CAD build for the part. Positions are in the model's coordinates, mm. A direction names the side the tool comes from. Give positions to 0.01 mm unless a question says otherwise; leave off trailing zeros. Write each loop counter-clockwise with the first axis right and the second up, starting at its lowest first coordinate (ties: lowest second). Pieces come first, ordered by that corner, then holes. Notation, with made-up numbers: (41.5, 30) - (54.5, 30) arc R17 ccw to (54.5, 58) - close; hole circle Ø11 at (54, 27). An arc over 180 degrees is marked (long way). Answer as a JSON object with one key per item and string values.
from build123d import *

# Parameters (mm, degrees)
BOSS_EXTRUDE1_DEPTH      = 1
BOSS_EXTRUDE1_DEPTH_BACK = 1
SKETCH1_R                = 45.5
SKETCH1_R_2              = 7.6
SKETCH1_R_3              = 4.774915174
BOSS_EXTRUDE2_DEPTH      = 1.5
BOSS_EXTRUDE2_DEPTH_BACK = 1.5
SKETCH1_3_R              = 47.5
SKETCH1_3_R_2            = 45.5
BOSS_EXTRUDE6_DEPTH      = 20
BOSS_EXTRUDE6_DEPTH_BACK = 60
SKETCH1_6_R              = 7.6
SKETCH1_6_R_2            = 6.9
CUT_EXTRUDE1_DEPTH       = 20


with BuildPart() as part:
    # Sketch1 → Boss-Extrude1 (new, two sides: drawn at the far end of the back side and taken through both)
    with BuildSketch(Plane.XY.offset(-BOSS_EXTRUDE1_DEPTH_BACK)):
        Circle(SKETCH1_R)
        with Locations((-26.162950904, -26.162950904)):
            Circle(SKETCH1_R_2, mode=Mode.SUBTRACT)
        with Locations((26.162950904, -26.162950904)):
            Circle(SKETCH1_R_2, mode=Mode.SUBTRACT)
        with Locations((26.162950904, 26.162950904)):
            Circle(SKETCH1_R_2, mode=Mode.SUBTRACT)
        with Locations((-26.162950904, 26.162950904)):
            Circle(SKETCH1_R_2, mode=Mode.SUBTRACT)
        Circle(SKETCH1_R_3, mode=Mode.SUBTRACT)
    extrude(amount=BOSS_EXTRUDE1_DEPTH + BOSS_EXTRUDE1_DEPTH_BACK)

    # Sketch1_3 → Boss-Extrude2 (add, two sides: drawn at the far end of the back side and taken through both)
    with BuildSketch(Plane.XY.offset(-BOSS_EXTRUDE2_DEPTH_BACK)):
        Circle(SKETCH1_3_R)
        Circle(SKETCH1_3_R_2, mode=Mode.SUBTRACT)
    extrude(amount=BOSS_EXTRUDE2_DEPTH + BOSS_EXTRUDE2_DEPTH_BACK)

    # Sketch1_6 → Boss-Extrude6 (add, two sides: drawn at the far end of the back side and taken through both)
    # profile 1 of 4: a face of its own
    with BuildSketch(Plane.XY.offset(-BOSS_EXTRUDE6_DEPTH_BACK)):
        with Locations((-26.162950904, 26.162950904)):
            Circle(SKETCH1_6_R)
        with Locations((-26.162950904, 26.162950904)):
            Circle(SKETCH1_6_R_2, mode=Mode.SUBTRACT)
    # profile 2 of 4: a face of its own
    with BuildSketch(Plane.XY.offset(-BOSS_EXTRUDE6_DEPTH_BACK)):
        with Locations((26.162950904, 26.162950904)):
            Circle(SKETCH1_6_R)
        with Locations((26.162950904, 26.162950904)):
            Circle(SKETCH1_6_R_2, mode=Mode.SUBTRACT)
    # profile 3 of 4: a face of its own
    with BuildSketch(Plane.XY.offset(-BOSS_EXTRUDE6_DEPTH_BACK)):
        with Locations((26.162950904, -26.162950904)):
            Circle(SKETCH1_6_R)
        with Locations((26.162950904, -26.162950904)):
            Circle(SKETCH1_6_R_2, mode=Mode.SUBTRACT)
    # profile 4 of 4: a face of its own
    with BuildSketch(Plane.XY.offset(-BOSS_EXTRUDE6_DEPTH_BACK)):
        with Locations((-26.162950904, -26.162950904)):
            Circle(SKETCH1_6_R)
        with Locations((-26.162950904, -26.162950904)):
            Circle(SKETCH1_6_R_2, mode=Mode.SUBTRACT)
    extrude(amount=BOSS_EXTRUDE6_DEPTH + BOSS_EXTRUDE6_DEPTH_BACK)

    # Sketch2 → Cut-Extrude1 (cut)
    with BuildSketch(Plane.XY.offset(20)):
        Polygon((-31.533797235, 30.40024079), (-30.967019012, 30.967019012), (-31.567102172, 31.567102172), (-32.073769026, 30.940212581), align=None)
        Polygon((-31.567102172, 31.567102172), (-30.967019012, 30.967019012), (-30.40024079, 31.533797235), (-30.940212581, 32.073769026), align=None)
        Polygon((32.073769026, 30.940212581), (31.533797235, 30.40024079), (30.40024079, 31.533797235), (30.940212581, 32.073769026), (31.567102172, 31.567102172), align=None)
        Polygon((30.940212581, -32.073769026), (30.40024079, -31.533797235), (31.533797235, -30.40024079), (32.073769026, -30.940212581), (31.567102172, -31.567102172), align=None)
        Polygon((-32.073769026, -30.940212581), (-31.533797235, -30.40024079), (-30.40024079, -31.533797235), (-30.940212581, -32.073769026), (-31.567102172, -31.567102172), align=None)
    extrude(amount=-CUT_EXTRUDE1_DEPTH, mode=Mode.SUBTRACT)


solid = part.part
Item 1: Probe line 1 (X direction, y = 27.5, z = -2); line 2 (Z direction, x = 29, y = -11); line 3 (X direction, y = 31, z = -27). List the from-to ranges inside material, lowest first. Write a range as from..to.
Entries:
{"line 1": "-33.64..-32.93, -19.39..-18.68, 18.68..19.39, 32.93..33.64", "line 2": "-1..1", "line 3": "-32.02..-31.08, -21.24..-20.3, 20.3..21.24, 31.08..32.02"}
Item 2: Cut at C-C (y = -3.5). Give the cut face in (x, z).
Entries:
{"outline": "(-47.37, -1.5) - (-45.37, -1.5) - (-45.37, -1) - (-3.25, -1) - (-3.25, 1) - (-45.37, 1) - (-45.37, 1.5) - (-47.37, 1.5) - close; (3.25, -1) - (45.37, -1) - (45.37, -1.5) - (47.37, -1.5) - (47.37, 1.5) - (45.37, 1.5) - (45.37, 1) - (3.25, 1) - close"}
Item 3: Mould opens along X. For faces 4 (the cylindrical face through (-10.3, -46.37, -0.02)), 5 (the cylindrical face through (32.744, -24.09, -20.56)), 6 (the cylindrical face through (32.744, 28.236, -20.56)), 7 (the flat face through (-25, 19, -60)) say: +X half, -X half, draft (parallel to the pull), parting line (faces both ways), or undercut.
Entries:
{"face 4": "parting line", "face 5": "undercut", "face 6": "undercut", "face 7": "draft"}
Item 4: Which spindle directions (+Z, -Z, +X, -X, +Y, -Y) get a long thin tool onto all of the face, cutting with end or side? Do faces 1 (the flat face through (28, -33, -60)), 2 (the cylindrical face through (21.02, -20.57, 10.37)), 3 (the cylindrical face through (-36.107, -27.686, -1.254)). Say none if no direction does.
Entries:
{"face 1": "-Z, +X, -X, +Y, -Y", "face 2": "+Z", "face 3": "-Z"}
Item 5: Flat gauge pins, fed straight in: P1, Ø4, axis at x = -24, z = -41.5, coming from the +Y side; P2, Ø1.5, axis at y = -28, z = -46, coming from the -X side; P3, Ø1.3, axis at x = 31, y = -31, coming from the +Z side. Where does each tip first touch, or does it go through?
Entries:
{"P1": "y = 33.76", "P2": "x = -33.68", "P3": "z = 0"}
Item 6: Cut at A-A (z = -34). Give the cut face in (x, y), and give its area (3 significant figures).
Entries:
{"outline": "circle Ø15.2 at (-26.16, -26.16); circle Ø15.2 at (-26.16, 26.16); circle Ø15.2 at (26.16, -26.16); circle Ø15.2 at (26.16, 26.16); hole circle Ø13.8 at (-26.16, -26.16); hole circle Ø13.8 at (-26.16, 26.16); hole circle Ø13.8 at (26.16, -26.16); hole circle Ø13.8 at (26.16, 26.16)", "area": "128 mm2"}
Item 7: Cut at D-D (y = 16). Give the cut face in (x, z).
Entries:
{"outline": "(-44.72, -1.5) - (-42.59, -1.5) - (-42.59, -1) - (42.59, -1) - (42.59, -1.5) - (44.72, -1.5) - (44.72, 1.5) - (42.59, 1.5) - (42.59, 1) - (-42.59, 1) - (-42.59, 1.5) - (-44.72, 1.5) - close"}
Item 8: Cut at B-B (x = 0). Give the cut face in (y, z), and give its area (3 significant figures).
Entries:
{"outline": "(-47.5, -1.5) - (-45.5, -1.5) - (-45.5, -1) - (-4.77, -1) - (-4.77, 1) - (-45.5, 1) - (-45.5, 1.5) - (-47.5, 1.5) - close; (4.77, -1) - (45.5, -1) - (45.5, -1.5) - (47.5, -1.5) - (47.5, 1.5) - (45.5, 1.5) - (45.5, 1) - (4.77, 1) - close", "area": "175 mm2"}
